Check sheet for the drawn part. Datum: minimum x, y, z corner. Units: mm. Give positions to 0.01 mm unless a question says otherwise; leave off trailing zeros. Order: outer loops, then holes, each group sorted by start corner. A loop starts at its lowest first (then second) coordinate and runs counter-clockwise, first axis right, second up. Notation, with made-up numbers: M 43.5,80.25 L 72.5,80.25 A25 ccw 72.5,114.25 Z; hole C 0,-21.5 d11. An arc over 180 degrees is marked long. Answer in a Markdown table with one row per item. Add a question column.
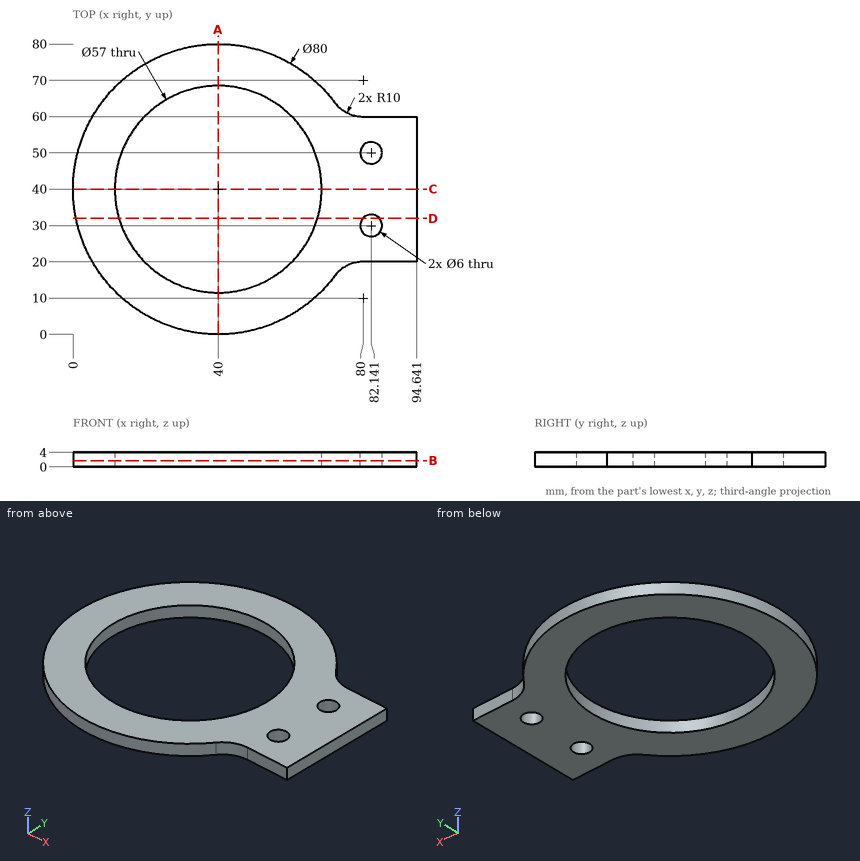
Q1. Cross-section at C-C (y = 40). Record the boundary of the cut face in (x, z).
Q2. Cross-section at B-B (z = 1.75). Record the boundary of the cut face in (x, y).
Q3. Go/stop test with flat-tipped pins: pin 1 (1.5 mm diameter, centred on y = 11, z = 3.5, fed in from -X); pin 2 (1.2 mm diameter, centred on x = 87, z = 2, fed in from +Y); pin 3 (2 mm diameter, centred on y = 55.5, z = 2, fed in from -X). Record where each tip stops, or that it passes through.
Q4. Cross-section at A-A (x = 40). Record the boundary of the cut face in (y, z), and give its area (3 significant figures).
Q5. Thickness scan on probe 1 along Y at (x, z) = (41, 0.95); probe 2 along X at (y, z) = (30, 1.9); probe 3 along Y at (x, z) = (80.5, 1.9). Record the ranges inside material, lowest first.
Q6. Cross-section at D-D (y = 32). Record the boundary of the cut face in (x, z), and give its area (3 significant figures).
Values follow:
| question | item | result |
|---|---|---|
| 1 | outline | M 0,0 L 11.5,0 L 11.5,4 L 0,4 Z; M 68.5,0 L 94.64,0 L 94.64,4 L 68.5,4 Z |
| 2 | outline | M 72,16 A10 cw 80,20 L 94.64,20 L 94.64,60 L 80,60 A10 cw 72,64 A40 ccw long Z; hole C 40,40 d57; hole C 82.14,30 d6; hole C 82.14,50 d6 |
| 3 | pin 1 | x = 11.68 |
| 3 | pin 2 | y = 60 |
| 3 | pin 3 | x = 2.72 |
| 4 | outline | M 0,0 L 11.5,0 L 11.5,4 L 0,4 Z; M 68.5,0 L 80,0 L 80,4 L 68.5,4 Z |
| 4 | area | 92.0 mm² |
| 5 | probe 1 | 0.01 to 11.52, 68.48 to 79.99 |
| 5 | probe 2 | 1.27 to 13.31, 66.69 to 79.14, 85.14 to 94.64 |
| 5 | probe 3 | 20 to 27.49, 32.51 to 47.49, 52.51 to 60 |
| 6 | outline | M 0.81,0 L 12.65,0 L 12.65,4 L 0.81,4 Z; M 67.35,0 L 79.9,0 L 79.9,4 L 67.35,4 Z; M 84.38,0 L 94.64,0 L 94.64,4 L 84.38,4 Z |
| 6 | area | 139 mm² |
